Design review of the part built by this model. Coordinates are the model's own, in mm. A direction names the side the tool comes from. Coordinates: 2 decimals unless noted, no trailing zeros. Write each loop counter-clockwise with the first axis right and the second up, starting at its lowest first coordinate (ties: lowest second). Pieces come first, ordered by that corner, then holes. Notation, with made-up numbers: (60, 74) - (103, 74) arc R19 cw to (103, 100) - close; hole circle Ø11 at (77.25, 40.25). An arc over 180 degrees is marked (long way). One line per item, written item: value.
from build123d import *

# Parameters (mm, degrees)
SKETCH1_W                    = 27
SKETCH1_H                    = 400
BASE_FLANGE1_DEPTH           = 2
EDGE_FLANGE1_STRIP_W         = 9.4732
EDGE_FLANGE1_STRIP_H         = 2
EDGE_FLANGE1_STRIP_CUT_DEPTH = 400
EDGE_FLANGE1_DEPTH           = 400
EDGE_FLANGE2_STRIP_W         = 9.4732
EDGE_FLANGE2_STRIP_H         = 2
EDGE_FLANGE2_STRIP_CUT_DEPTH = 400
EDGE_FLANGE2_DEPTH           = 400
EDGE_FLANGE3_STRIP_W         = 9.4732
EDGE_FLANGE3_STRIP_H         = 2
EDGE_FLANGE3_STRIP_CUT_DEPTH = 400
EDGE_FLANGE3_DEPTH           = 400
EDGE_FLANGE4_STRIP_W         = 9.4732
EDGE_FLANGE4_STRIP_H         = 2
EDGE_FLANGE4_STRIP_CUT_DEPTH = 400
EDGE_FLANGE4_DEPTH           = 400
SKETCH18_R                   = 3
CUT_EXTRUDE1_DEPTH           = 219.021214564
SKETCH19_R                   = 3
CUT_EXTRUDE2_DEPTH           = 219.021214564


# Sheet-metal steps are written as plain solids
with BuildPart() as part:
    # Sketch1 → Base-Flange1 (new body)
    with BuildSketch(Plane(origin=(0, 0, 0), x_dir=(1, 0, 0), z_dir=(0, 1, 0))):
        Rectangle(SKETCH1_W, SKETCH1_H)
    extrude(amount=-BASE_FLANGE1_DEPTH)

    # Edge-Flange1 strip (across the edge) → Edge-Flange1 strip cut (cut)
    with BuildSketch(Plane(origin=(13.5, 0, 200), x_dir=(-1, 0, 0), z_dir=(0, 0, -1))):
        with Locations((-2, -1)):
            Rectangle(EDGE_FLANGE1_STRIP_W, EDGE_FLANGE1_STRIP_H)
    extrude(amount=EDGE_FLANGE1_STRIP_CUT_DEPTH, mode=Mode.SUBTRACT)

    # Edge-Flange1 section (across the edge) → Edge-Flange1 (add)
    with BuildSketch(Plane(origin=(13.5, 0, 200), x_dir=(-1, 0, 0), z_dir=(0, 0, -1))):
        with BuildLine():
            Line((0, 0.7366), (0, 33))
            Line((0, 33), (2, 33))
            Line((2, 33), (2, 0.7366))
            ThreePointArc((2, 0.7366), (2.215745145, 0.215745145), (2.7366, 0))
            Line((2.7366, 0), (2.7366, -2))
            ThreePointArc((2.7366, -2), (0.801531583, -1.198468417), (0, 0.7366))
        make_face()
    extrude(amount=EDGE_FLANGE1_DEPTH)

    # Edge-Flange2 strip (across the edge) → Edge-Flange2 strip cut (cut)
    with BuildSketch(Plane(origin=(11.5, 33, 200), x_dir=(0, -1, 0), z_dir=(0, 0, -1))):
        with Locations((-2, -1)):
            Rectangle(EDGE_FLANGE2_STRIP_W, EDGE_FLANGE2_STRIP_H)
    extrude(amount=EDGE_FLANGE2_STRIP_CUT_DEPTH, mode=Mode.SUBTRACT)

    # Edge-Flange2 section (across the edge) → Edge-Flange2 (add)
    with BuildSketch(Plane(origin=(11.5, 33, 200), x_dir=(0, -1, 0), z_dir=(0, 0, -1))):
        with BuildLine():
            Line((0, 0.7366), (0, 21))
            Line((0, 21), (2, 21))
            Line((2, 21), (2, 0.7366))
            ThreePointArc((2, 0.7366), (2.215745145, 0.215745145), (2.7366, 0))
            Line((2.7366, 0), (2.7366, -2))
            ThreePointArc((2.7366, -2), (0.801531583, -1.198468417), (0, 0.7366))
        make_face()
    extrude(amount=EDGE_FLANGE2_DEPTH)

    # Edge-Flange3 strip (across the edge) → Edge-Flange3 strip cut (cut)
    with BuildSketch(Plane(origin=(-9.5, 33, -200), x_dir=(1, 0, 0), z_dir=(0, 0, 1))):
        with Locations((-2, -1)):
            Rectangle(EDGE_FLANGE3_STRIP_W, EDGE_FLANGE3_STRIP_H)
    extrude(amount=EDGE_FLANGE3_STRIP_CUT_DEPTH, mode=Mode.SUBTRACT)

    # Edge-Flange3 section (across the edge) → Edge-Flange3 (add)
    with BuildSketch(Plane(origin=(-9.5, 33, -200), x_dir=(1, 0, 0), z_dir=(0, 0, 1))):
        with BuildLine():
            Line((0, 0.7366), (0, 8))
            Line((0, 8), (2, 8))
            Line((2, 8), (2, 0.7366))
            ThreePointArc((2, 0.7366), (2.215745145, 0.215745145), (2.7366, 0))
            Line((2.7366, 0), (2.7366, -2))
            ThreePointArc((2.7366, -2), (0.801531583, -1.198468417), (0, 0.7366))
        make_face()
    extrude(amount=EDGE_FLANGE3_DEPTH)

    # Edge-Flange4 strip (across the edge) → Edge-Flange4 strip cut (cut)
    with BuildSketch(Plane(origin=(-7.5, 41, -200), x_dir=(0, -1, 0), z_dir=(0, 0, 1))):
        with Locations((-2, -1)):
            Rectangle(EDGE_FLANGE4_STRIP_W, EDGE_FLANGE4_STRIP_H)
    extrude(amount=EDGE_FLANGE4_STRIP_CUT_DEPTH, mode=Mode.SUBTRACT)

    # Edge-Flange4 section (across the edge) → Edge-Flange4 (add)
    with BuildSketch(Plane(origin=(-7.5, 41, -200), x_dir=(0, -1, 0), z_dir=(0, 0, 1))):
        with BuildLine():
            Line((0, 0.7366), (0, 39))
            Line((0, 39), (2, 39))
            Line((2, 39), (2, 0.7366))
            ThreePointArc((2, 0.7366), (2.215745145, 0.215745145), (2.7366, 0))
            Line((2.7366, 0), (2.7366, -2))
            ThreePointArc((2.7366, -2), (0.801531583, -1.198468417), (0, 0.7366))
        make_face()
    extrude(amount=EDGE_FLANGE4_DEPTH)

    # Mirror1: part across plane


with BuildPart() as part_1:
    add(part.part)
    add(part.part.mirror(Plane(origin=(31.5, 41, -200), x_dir=(0, 0, 1), z_dir=(-1, 0, 0))))

    # Sketch18 → Cut-Extrude1 (cut, through all)
    with BuildSketch(Plane(origin=(0, 0, 0), x_dir=(1, 0, 0), z_dir=(0, 1, 0))):
        with Locations(Location((6.5, 180, 0), (0, 0, 270))):
            Circle(SKETCH18_R)
        with Locations(Location((56.5, 130, 0), (0, 0, 270))):
            Circle(SKETCH18_R)
        with Locations(Location((56.5, 180, 0), (0, 0, 270))):
            Circle(SKETCH18_R)
        with Locations(Location((6.5, 130, 0), (0, 0, 270))):
            Circle(SKETCH18_R)
    extrude(amount=-CUT_EXTRUDE1_DEPTH, mode=Mode.SUBTRACT)

    # Sketch19 → Cut-Extrude2 (cut, through all)
    with BuildSketch(Plane(origin=(0, 0, 0), x_dir=(1, 0, 0), z_dir=(0, 1, 0))):
        with Locations(Location((56.5, -142.75, 0), (0, 0, 270))):
            Circle(SKETCH19_R)
        with Locations(Location((56.5, -52.75, 0), (0, 0, 270))):
            Circle(SKETCH19_R)
        with Locations(Location((56.5, 37.25, 0), (0, 0, 270))):
            Circle(SKETCH19_R)
        with Locations(Location((6.5, 37.25, 0), (0, 0, 270))):
            Circle(SKETCH19_R)
        with Locations(Location((6.5, -52.75, 0), (0, 0, 270))):
            Circle(SKETCH19_R)
        with Locations(Location((6.5, -142.75, 0), (0, 0, 270))):
            Circle(SKETCH19_R)
    extrude(amount=-CUT_EXTRUDE2_DEPTH, mode=Mode.SUBTRACT)


solid = part_1.part
1. Mouldability with a two-part tool opening along Y and no side actions: class faces 1 (the face through (-2, 0, -3)), 2 (the face through (32, 41, -3)), 3 (the face through (51.5, 16, 3)), 4 (the face through (65, -2, -3)) as released by +Y, released by -Y, zero draft, split by the parting line, or undercut.
Answer block:
face 1: undercut
face 2: released by +Y
face 3: undercut
face 4: released by -Y
2. For faces 5 (the face through (65, 0, -3)), 6 (the face through (61, 33, 3)), 7 (the face through (13.5, 15, 3)), list the 3-axis set-ups (+Z, -Z, +X, -X, +Y, -Y) from which the entire face can be reached by the end or side of a thin tool; tool diameter is ignored.
Answer block:
face 5: +Z, -Z, +X
face 6: +Z, -Z
face 7: +Z, -Z, -Y
3. Consider section A-A, the plane y = 5. Write out the cut boundary in (x, z), then the cut area to 3 significant figures.
Answer block:
outline: (11.5, -200) - (13.5, -200) - (13.5, 200) - (11.5, 200) - close; (49.5, -200) - (51.5, -200) - (51.5, 200) - (49.5, 200) - close
area: 1,600 mm^2
4. Wall thickness on line 1 along Y through (x, z) = (10, -168); line 2 along Z through (x, y) = (6, -1); line 3 along X through (y, z) = (38.5, -42): over which ranges is each line inside the solid? List them lowest first.
Answer block:
line 1: y = -2 to 0, 31 to 33, 39 to 41
line 2: z = -200 to -182.96, -177.04 to -132.96, -127.04 to -40.21, -34.29 to 49.79, 55.71 to 139.79, 145.71 to 200
line 3: x = -9.49 to -7.46, 70.46 to 72.49
5. Insertion check: pin 1 Ø15 at (y, z) = (20, 36.5) entering from -X; pin 2 Ø5 at (y, z) = (37, 73.5) entering from -X; pin 3 Ø5 at (y, z) = (35, 35.5) entering from +X; pin 4 Ø10 at (x, y) = (27.5, 32) entering from +Z. Each pin has a flat end and moves straight along its axis. Give the tip position at first contact, or say it passes through.
Answer block:
pin 1: stops at x = 11.5
pin 2: stops at x = -9.5
pin 3: stops at x = 72.5
pin 4: passes through
